from build123d import *

# Parameters (mm, degrees)
F0_R     = 30
F1_DEPTH = 4
F2_R     = 6
F3_DEPTH = 6
F4_R     = 1.5
F5_DEPTH = 12.5
F6_W     = 3
F6_H     = 4.6
F7_DEPTH = 9.4


with BuildPart() as f1:
    # F0 (on Top) → F1 (new body)
    with BuildSketch(Plane.XY):
        Circle(F0_R)
    extrude(amount=F1_DEPTH)

    # F2 (on face) → F3 (join)
    with BuildSketch(Plane.XY.offset(4)):
        Circle(F2_R)
    extrude(amount=F3_DEPTH)

    # F4 (on Front) → F5 (cut, symmetric)
    with BuildSketch(Plane.XZ):
        with Locations((0, 7)):
            Circle(F4_R)
    extrude(amount=F5_DEPTH, both=True, mode=Mode.SUBTRACT)

    # F6 (on face) → F7 (cut)
    with BuildSketch(Plane.XY.offset(10)):
        with BuildLine():
            ThreePointArc((-1.5, -2.3), (0, -2.745184), (1.5, -2.3))
            Line((1.5, -2.3), (-1.5, -2.3))
        make_face()
        Rectangle(F6_W, F6_H)
        with BuildLine():
            Line((-1.5, 2.3), (1.5, 2.3))
            ThreePointArc((1.5, 2.3), (0, 2.745906), (-1.5, 2.3))
        make_face()
    extrude(amount=-F7_DEPTH, mode=Mode.SUBTRACT)


solid = f1.part
CAD build for the part. Positions are in the model's coordinates, mm. A direction names the side the tool comes from. Round coordinates to 2 decimals unless told otherwise and drop trailing zeros. Write each loop counter-clockwise with the first axis right and the second up, starting at its lowest first coordinate (ties: lowest second). Pieces come first, ordered by that corner, then holes.
(1) Slice it at A-A, the plane x = 0. Write the cut outline in (y, z).
(2) Mould opens along X. For faces 1 (the face through (0.022, 2.746, 3.134)), 2 (the face through (6.2, 0.4, 4)), 3 (the face through (-29.97, 1.32, 1.97)), 4 (the face through (-0.325, 4.127, 5.536)) say: pulls with the +X half, pulls with the -X half, needs draft (parallel to the pull), parting line crosses it, or undercut.
(3) Probe line 1 along Z through (x, y) = (0, -4); line 2 along Z through (x, y) = (-21.5, 13.5); line 3 along X through (y, z) = (3.95, 7). List the from-to ranges inside material, lowest first.
(4) Slice it at B-B, the plane y = 0. Write the cut outline in (x, z).
(5) Drop flat-ended pins along their axis: P1, Ø4, axis at x = 0, z = 7, coming from the +Y side; P2, Ø5, axis at x = -10, y = 5, coming from the +Z side; P3, Ø6, axis at y = -4, z = 3, coming from the +X side. Give the stop position or say it passes through.
(6) 3-axis set-ups, long thin cutter, end or side, ignore diameter. For faces 5 (the face through (5.54, -2.3, 6.96)), 6 (the face through (1.386, -4.179, 6.425)): which of +Z, -Z, +X, -X, +Y, -Y reach the whole face in a straight line?
(7) Slice it at C-C, the plane z = 1.75. Write the cut outline in (x, y), and give its area (3 significant figures).
(8) Slice it at D-D, the plane x = 24. Write the cut outline in (y, z).
From the geometry:
1. outline: (-30, 0) - (30, 0) - (30, 4) - (6, 4) - (6, 5.5) - (2.75, 5.5) - (2.75, 0.6) - (-2.75, 0.6) - (-2.75, 5.5) - (-6, 5.5) - (-6, 4) - (-30, 4) - close; (-6, 8.5) - (-2.75, 8.5) - (-2.75, 10) - (-6, 10) - close; (2.75, 8.5) - (6, 8.5) - (6, 10) - (2.75, 10) - close
2. face 1: undercut
2. face 2: needs draft
2. face 3: parting line crosses it
2. face 4: undercut
3. line 1: z = 0 to 5.5, 8.5 to 10
3. line 2: z = 0 to 4
3. line 3: x = -4.52 to -1.5, 1.5 to 4.52
4. outline: (-30, 0) - (30, 0) - (30, 4) - (6, 4) - (6, 10) - (1.5, 10) - (1.5, 0.6) - (-1.5, 0.6) - (-1.5, 10) - (-6, 10) - (-6, 4) - (-30, 4) - close
5. P1: stops at y = 6
5. P2: stops at z = 4
5. P3: stops at x = 29.98
6. face 5: +Z
6. face 6: +Y, -Y
7. outline: circle Ø60 at (0, 0); hole (-1.5, -2.3) arc R2.75 ccw to (1.5, -2.3) - (1.5, 2.3) arc R2.75 ccw to (-1.5, 2.3) - close
7. area: 2,810 mm2
8. outline: (-18, 0) - (18, 0) - (18, 4) - (-18, 4) - close
